Source: CAD feature listing. Evaluate the final solid. Frame: model axes, mm. Face numbers are marked on the shaded views. A direction names the side the tool comes from. Give positions to 0.01 mm unless a question says otherwise; leave off trailing zeros. Order: outer loops, then holes, each group sorted by start corner. A loop starts at its lowest first (then second) coordinate and runs counter-clockwise, first axis right, second up. Notation, with made-up numbers: M 33.5,-19 L 90.5,-19 A12 cw 90.5,-1 Z; hole C 56.25,-19.5 d9. An arc over 180 degrees is marked long. Return JSON: item names as keys, results as strings.
from build123d import *

# Parameters (mm, degrees)
F0_W          = 5.842
F0_H          = 12.7
F0_R          = 3.175
F2_DEPTH      = 3.175
F3_R          = 1.524
F4_DEPTH      = 6.35
F4_DEPTH_BACK = 1.27


with BuildPart() as f1:
    # F0 (on Front) → F1 (revolve)
    with BuildSketch(Plane.XZ):
        Polygon((5.842, 12.7), (5.842, 0), (66.294, 0), (66.294, 12.7), (56.134, 12.7), (56.134, 10.16), (10.16, 10.16), (10.16, 12.7), align=None)
        with Locations((2.921, 6.35)):
            Rectangle(F0_W, F0_H)
    revolve(axis=Axis((33.147, 0, 0), (-1, 0, 0)))

    # F0 (on Front) → F2 (join, symmetric)
    with BuildSketch(Plane.XZ):
        with Locations((2.921, 6.35)):
            Rectangle(F0_W, F0_H)
        with BuildLine():
            Line((-0.9398, 0), (0, 0))
            Line((0, 0), (0, 12.7))
            Line((0, 12.7), (5.842, 12.7))
            Line((5.842, 12.7), (5.842, 15.24))
            Line((5.842, 15.24), (-0.508, 15.24))
            Line((-0.508, 15.24), (-10.88063, 3.847543))
            ThreePointArc((-10.88063, 3.847543), (-4.591961, 5.329721), (-0.9398, 0))
        make_face()
        with BuildLine():
            ThreePointArc((-8.182663, -5.506983), (-3.195791, -4.549339), (-0.9398, 0))
            ThreePointArc((-0.9398, 0), (-4.591961, 5.329721), (-10.88063, 3.847543))
            ThreePointArc((-10.88063, 3.847543), (-12.145978, -1.583727), (-8.182663, -5.506983))
        make_face()
        with Locations((-6.6548, 0)):
            Circle(F0_R, mode=Mode.SUBTRACT)
    extrude(amount=F2_DEPTH, both=True)

    # F3 (on face) → F4 (join, two sides)
    with BuildSketch(Plane.YZ.offset(66.294)) as f4_sk:
        with BuildLine():
            ThreePointArc((-5.08, 0), (0, -5.08), (5.08, 0))
            ThreePointArc((5.08, 0), (0, 5.08), (-5.08, 0))
        make_face()
        Circle(F3_R, mode=Mode.SUBTRACT)
        with BuildLine():
            ThreePointArc((-5.08, 0), (0, 5.08), (5.08, 0))
            Line((5.08, 0), (5.08, 15.24))
            Line((5.08, 15.24), (-5.08, 15.24))
            Line((-5.08, 15.24), (-5.08, 0))
        make_face()
    extrude(amount=F4_DEPTH)
    extrude(f4_sk.sketch, amount=-F4_DEPTH_BACK)


solid = f1.part
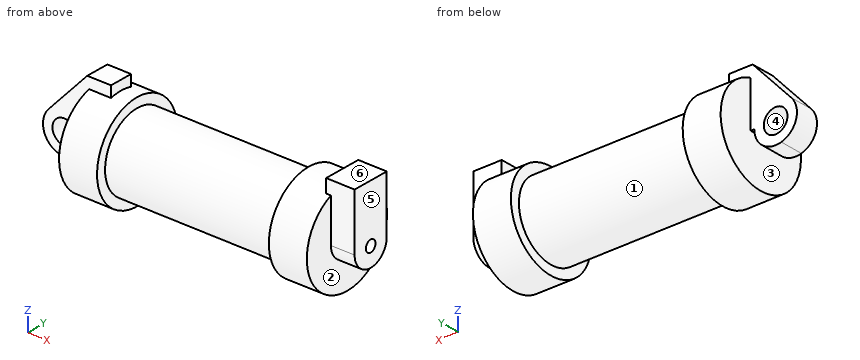
1. First-contact query: pin 1 (4 mm diameter, centred on x = 48, z = -9.5, fed in from -Y); pin 2 (5.5 mm diameter, centred on x = -1.5, z = 6, fed in from -Y); pin 3 (2.5 mm diameter, centred on x = 67, z = 9.5, fed in from -Y). Flat tips, straight axial feed; report the tip coordinate or a pass-through.
Evaluation:
{"pin 1": "stops at y = -6.85", "pin 2": "stops at y = -12.15", "pin 3": "stops at y = -9.46"}
2. Set-up query: the marked faces 1, 2 and 3. Return all of +Z, -Z, +X, -X, +Y, -Y with unobstructed straight access to the full face (end or side cutting, diameter ignored); none if empty.
Evaluation:
{"face 1": "none", "face 2": "-Z, +X", "face 3": "-Z"}
3. Ray query, probe 1 along X at (y, z) = (-10.25, -3); probe 2 along Z at (x, y) = (71, 0); probe 3 along X at (y, z) = (2.25, 11.75). Return the intervals inside material, ascending.
Evaluation:
{"probe 1": "x = 0 to 10.16, 56.13 to 66.29", "probe 2": "z = -5.08 to -1.52, 1.52 to 15.24", "probe 3": "x = -3.69 to 10.16, 56.13 to 72.64"}
4. Section query B-B (z = 13.5). Return loops of the section in (x, y) (3 decimals).
Evaluation:
{"outline": "M -2.092,-3.175 L 5.842,-3.175 L 5.842,3.175 L -2.092,3.175 Z; M 65.024,-5.08 L 72.644,-5.08 L 72.644,5.08 L 65.024,5.08 Z"}
5. Section query C-C (z = -0.75). Return loops of the section in (x, y) (3 decimals), then the cut area to 3 significant figures.
Evaluation:
{"outline": "M -12.32,-3.175 L -9.74,-3.175 L -9.74,3.175 L -12.32,3.175 Z; M -3.57,-3.175 L -0.989,-3.175 L -0.989,3.175 L -3.57,3.175 Z; M 0,-12.678 L 10.16,-12.678 L 10.16,-10.132 L 56.134,-10.132 L 56.134,-12.678 L 66.294,-12.678 L 66.294,-5.024 L 72.644,-5.024 L 72.644,-1.327 L 66.294,-1.327 L 66.294,1.327 L 72.644,1.327 L 72.644,5.024 L 66.294,5.024 L 66.294,12.678 L 56.134,12.678 L 56.134,10.132 L 10.16,10.132 L 10.16,12.678 L 0,12.678 Z", "area": "1,530 mm^2"}
6. Section query A-A (y = 0). Return loops of the section in (x, z) (3 decimals), then the cut area to 3 significant figures.
Evaluation:
{"outline": "M -10.881,3.848 A5.715 ccw long -0.94,0 L 0,0 L 0,-12.7 L 10.16,-12.7 L 10.16,-10.16 L 56.134,-10.16 L 56.134,-12.7 L 66.294,-12.7 L 66.294,-5.08 L 72.644,-5.08 L 72.644,-1.524 L 66.294,-1.524 L 66.294,1.524 L 72.644,1.524 L 72.644,15.24 L 65.024,15.24 L 65.024,12.7 L 56.134,12.7 L 56.134,10.16 L 10.16,10.16 L 10.16,12.7 L 5.842,12.7 L 5.842,15.24 L -0.508,15.24 Z; hole C -6.655,0 d6.35", "area": "1,710 mm^2"}
7. Section query D-D (z = 7). Return loops of the section in (x, y) (3 decimals).
Evaluation:
{"outline": "M -8.01,-3.175 L 0,-3.175 L 0,-10.597 L 10.16,-10.597 L 10.16,-7.364 L 56.134,-7.364 L 56.134,-10.597 L 66.294,-10.597 L 66.294,-5.08 L 72.644,-5.08 L 72.644,5.08 L 66.294,5.08 L 66.294,10.597 L 56.134,10.597 L 56.134,7.364 L 10.16,7.364 L 10.16,10.597 L 0,10.597 L 0,3.175 L -8.01,3.175 Z"}
8. Draft query along X for the marked faces 4, 5 and 6. Return one class per face: pulls with the +X half, pulls with the -X half, needs draft (parallel to the pull), parting line crosses it, or undercut.
Evaluation:
{"face 4": "undercut", "face 5": "pulls with the +X half", "face 6": "needs draft"}
